Geometry check sheet. Reference: the model listing, model coordinates, mm. A direction names the side the tool comes from. Give positions to 0.01 mm unless a question says otherwise; leave off trailing zeros. Loops run counter-clockwise (first coordinate to the right, second up) from the corner with the lowest first, then second, coordinate; pieces in that order, holes last. Notation, with made-up numbers: (52.5, 85.25) -> (94.5, 85.25) arc R14 ccw to (94.5, 92.25) -> close; hole circle Ø7 at (68.5, 83.5). An arc over 180 degrees is marked (long way). One line per question, with ' | ' between items.
Autodesk Inventor part; units mm, degrees
ref_plane "YZ Plane" through (0, 0, 0) normal (1, 0, 0) x (0, 1, 0)
ref_plane "XZ Plane" through (0, 0, 0) normal (0, 1, 0) x (-1, 0, 0)
ref_plane "XY Plane" through (0, 0, 0) normal (0, 0, 1) x (1, 0, 0)
sketch "スケッチ1" plane through (0, 0, 0) normal (0, 0, 1) x (1, 0, 0)
  line L0 (16, -16) -> (-16, -16)
  line L1 (-16, -16) -> (-16, 16)
  line L2 (-16, 16) -> (16, 16)
  line L3 (16, 16) -> (16, -16)
  line L4 (16, -16) -> (-16, 16) construction
  line L5 (-16, -16) -> (16, 16) construction
  line L6 (14.4, 14.4) -> (-14.4, 14.4)
  line L7 (-14.4, 14.4) -> (-14.4, -14.4)
  line L8 (-14.4, -14.4) -> (14.4, -14.4)
  line L9 (14.4, -14.4) -> (14.4, 14.4)
  point P0 (0, 0)
  dimension "d0" = 32
  dimension "d1" = 32
  dimension "d2" = 1.6
extrude "押し出し1" add sketch "スケッチ1" along normal mid plane 200
sketch "スケッチ3" plane through (16, -16, 100) normal (1, 0, 0) x (0, 0, -1)
  circle A0 centre (100, 16) radius 7.5
  dimension "d7" = 15
extrude "押し出し2" cut sketch "スケッチ3" against normal blind 30
chamfer "面取り2" distance 32 angle 45 1 edges at (16, 0, 100)
chamfer "面取り3" distance 32 angle 45 1 edges at (16, 0, -100)
properties part number "Pipe3"
Item 1: Sectioned sample at A-A (y = 0). Record the cut outline in (x, z), plus the area to 3 significant figures.
Result:
outline: (-16, -100) -> (-14.4, -98.4) -> (-14.4, 98.4) -> (-16, 100) -> close; (14.4, -69.6) -> (16, -68) -> (16, -7.5) -> (14.4, -7.5) -> close; (14.4, 7.5) -> (16, 7.5) -> (16, 68) -> (14.4, 69.6) -> close | area: 514 mm2
Item 2: Release check for a two-part mould opening along Y. For faces 1 (the face through (0, 14.4, -1)), 2 (the face through (16, 11, -1)), 3 (the face through (0, 16, -1)), 4 (the face through (15.211, 0.33, 7.493)) record: pulls with the +Y half, pulls with the -Y half, needs draft (parallel to the pull), parting line crosses it, or undercut.
Result:
face 1: undercut | face 2: needs draft | face 3: pulls with the +Y half | face 4: undercut
Item 3: Sectioned sample at C-C (z = 0). Record the cut outline in (x, y).
Result:
outline: (-16, -16) -> (16, -16) -> (16, -7.5) -> (14.4, -7.5) -> (14.4, -14.4) -> (-14.4, -14.4) -> (-14.4, 14.4) -> (14.4, 14.4) -> (14.4, 7.5) -> (16, 7.5) -> (16, 16) -> (-16, 16) -> close
Item 4: Sectioned sample at B-B (x = -1.5). Record the cut outline in (y, z), plus the area to 3 significant figures.
Result:
outline: (-16, -85.5) -> (-14.4, -85.5) -> (-14.4, 85.5) -> (-16, 85.5) -> close; (14.4, -85.5) -> (16, -85.5) -> (16, 85.5) -> (14.4, 85.5) -> close | area: 547 mm2
Item 5: Sectioned sample at D-D (y = 10). Record the cut outline in (x, z).
Result:
outline: (-16, -100) -> (-14.4, -98.4) -> (-14.4, 98.4) -> (-16, 100) -> close; (14.4, -69.6) -> (16, -68) -> (16, 68) -> (14.4, 69.6) -> close
Item 6: Set-up check for faces 5 (the face through (-14.4, 0, -1)), 6 (the face through (-1, -15, 85)): record each of +Z, -Z, +X, -X, +Y, -Y from which the full face is reachable in a straight line by a thin tool's end or side.
Result:
face 5: +Z, -Z | face 6: +Z, +X, +Y, -Y
Item 7: Depth check by flat-ended pin: pin 1 Ø4 at (y, z) = (8.5, 75) entering from +X. Enter the tip coordinate at first touch or a pass-through.
Result:
pin 1: x = -14.4
Item 8: Scan lines: probe 1 along X at (y, z) = (12.5, -6.5); probe 2 along Y at (x, z) = (15.7, 0). Record each from-to range of solid material in increasing order.
Result:
probe 1: -16 to -14.4, 14.4 to 16 | probe 2: -16 to -7.5, 7.5 to 16
